from build123d import *

# Parameters (mm, degrees)
SKETCH_1_W          = 4.5
SKETCH_1_H          = 4.5
SKETCH_1_R          = 1.5
EXTRUDE_1_DEPTH     = 2.5
EXTRUDE_1_2_DEPTH   = 2.5
EXTRUDE_1_3_DEPTH   = 2.5
EXTRUDE_1_4_DEPTH   = 2.5
SKETCH_2_W          = 3
SKETCH_2_H          = 65
EXTRUDE_2_DEPTH     = 40
SKETCH_3_W          = 59
SKETCH_3_H          = 40
SKETCH_3_R          = 1
SKETCH_3_R_2        = 1.5
SKETCH_3_W_2        = 32
SKETCH_3_H_2        = 32
EXTRUDE_4_DEPTH     = 2.5
EXTRUDE_5_DEPTH     = 3
EXTRUDE_6_DEPTH     = 3
SKETCH_9_W          = 65
SKETCH_9_H          = 70.660654221
EXTRUDE_8_DEPTH     = 1.8
SKETCH_12_R         = 1
SKETCH_12_W         = 32
SKETCH_12_H         = 32
CUT_EXTRUDE_2_DEPTH = 65
CUT_EXTRUDE_6_DEPTH = 65
SKETCH_14_R         = 1.5
CUT_EXTRUDE_8_DEPTH = 1.8


with BuildPart() as part:
    # Sketch 1 → Extrude 1 (new body)
    with BuildSketch(Plane(origin=(0, 0, 0), x_dir=(1, 0, 0), z_dir=(0, 1, 0))):
        with Locations((-34.75, -30.25)):
            Rectangle(SKETCH_1_W, SKETCH_1_H)
        with Locations(Location((-34.75, -30.25, 0), (0, 0, 270))):
            Circle(SKETCH_1_R, mode=Mode.SUBTRACT)
    extrude(amount=EXTRUDE_1_DEPTH)



with BuildPart() as body_2:
    # Sketch 1 → Extrude 1 2 (new body)
    with BuildSketch(Plane(origin=(0, 0, 0), x_dir=(1, 0, 0), z_dir=(0, 1, 0))):
        with Locations((34.75, -30.25)):
            Rectangle(SKETCH_1_W, SKETCH_1_H)
        with Locations(Location((34.75, -30.25, 0), (0, 0, 270))):
            Circle(SKETCH_1_R, mode=Mode.SUBTRACT)
    extrude(amount=EXTRUDE_1_2_DEPTH)


with BuildPart() as body_3:
    # Sketch 1 → Extrude 1 3 (new body)
    with BuildSketch(Plane(origin=(0, 0, 0), x_dir=(1, 0, 0), z_dir=(0, 1, 0))):
        with Locations((34.75, 30.25)):
            Rectangle(SKETCH_1_W, SKETCH_1_H)
        with Locations(Location((34.75, 30.25, 0), (0, 0, 270))):
            Circle(SKETCH_1_R, mode=Mode.SUBTRACT)
    extrude(amount=EXTRUDE_1_3_DEPTH)


with BuildPart() as body_4:
    # Sketch 1 → Extrude 1 4 (new body)
    with BuildSketch(Plane(origin=(0, 0, 0), x_dir=(1, 0, 0), z_dir=(0, 1, 0))):
        with Locations((-34.75, 30.25)):
            Rectangle(SKETCH_1_W, SKETCH_1_H)
        with Locations(Location((-34.75, 30.25, 0), (0, 0, 270))):
            Circle(SKETCH_1_R, mode=Mode.SUBTRACT)
    extrude(amount=EXTRUDE_1_4_DEPTH)


with BuildPart() as part_1:
    add(part.part)

    add(body_2.part)  # Extrude 2 merges body 2

    add(body_3.part)  # Extrude 2 merges body 3

    add(body_4.part)  # Extrude 2 merges body 4
    # Sketch 2 → Extrude 2 (add)
    with BuildSketch(Plane(origin=(0, 0, 0), x_dir=(-1, 0, 0), z_dir=(0, -1, 0))):
        with Locations((31, 0)):
            Rectangle(SKETCH_2_W, SKETCH_2_H)
        with Locations((-31, 0)):
            Rectangle(SKETCH_2_W, SKETCH_2_H)
    extrude(amount=-EXTRUDE_2_DEPTH)

    # Sketch 5 → Extrude 5 (add)
    with BuildSketch(Plane.ZY.offset(32.5)):
        Polygon((32.5, 40), (-19.677687078, 62.148114133), (-32.543475158, 67.609317163), (-32.5, 40), align=None)
    extrude(amount=-EXTRUDE_5_DEPTH)

    # Sketch 8 → Extrude 6 (add)
    with BuildSketch(Plane(origin=(32.5, 0, 0), x_dir=(0, 0, -1), z_dir=(1, 0, 0))):
        Polygon((-32.5, 40), (32.5, 40), (32.543475158, 67.609317163), align=None)
    extrude(amount=-EXTRUDE_6_DEPTH)



with BuildPart() as body_2_2:
    # Sketch 3 → Extrude 4 (new body)
    with BuildSketch(Plane.XY.offset(32.5)):
        with Locations((0, 20)):
            Rectangle(SKETCH_3_W, SKETCH_3_H)
        with Locations((-17.5, 37.5)):
            Circle(SKETCH_3_R, mode=Mode.SUBTRACT)
        with Locations((17.5, 37.5)):
            Circle(SKETCH_3_R, mode=Mode.SUBTRACT)
        with Locations((17.5, 2.5)):
            Circle(SKETCH_3_R, mode=Mode.SUBTRACT)
        with Locations((-17.5, 2.5)):
            Circle(SKETCH_3_R, mode=Mode.SUBTRACT)
        with Locations((-22.5, 20)):
            Circle(SKETCH_3_R_2, mode=Mode.SUBTRACT)
        with Locations((22.5, 20)):
            Circle(SKETCH_3_R_2, mode=Mode.SUBTRACT)
        with Locations((0, 20)):
            Rectangle(SKETCH_3_W_2, SKETCH_3_H_2, mode=Mode.SUBTRACT)
    extrude(amount=-EXTRUDE_4_DEPTH)


with BuildPart() as part_2:
    add(part_1.part)

    add(body_2_2.part)  # Extrude 8 merges body 2 2
    # Sketch 9 → Extrude 8 (add)
    with BuildSketch(Plane(origin=(0, 45.582439165, 19.348597487), x_dir=(1, 0, 0), z_dir=(0, 0.9205048534524402, 0.3907311284892746))):
        with Locations((0, 21.043164513)):
            Rectangle(SKETCH_9_W, SKETCH_9_H)
    extrude(amount=-EXTRUDE_8_DEPTH)

    # Sketch 12 → Cut-Extrude 2 (cut)
    with BuildSketch(Plane.ZY.offset(32.5)):
        with Locations((-17.5, 37.5)):
            Circle(SKETCH_12_R)
        with Locations((17.5, 37.5)):
            Circle(SKETCH_12_R)
        with Locations((17.5, 2.5)):
            Circle(SKETCH_12_R)
        with Locations((-17.5, 2.5)):
            Circle(SKETCH_12_R)
        with Locations((0, 20)):
            Rectangle(SKETCH_12_W, SKETCH_12_H)
    extrude(amount=-CUT_EXTRUDE_2_DEPTH, mode=Mode.SUBTRACT)

    # Sketch 13 → Cut-Extrude 6 (cut)
    with BuildSketch(Plane(origin=(32.5, 0, 0), x_dir=(0, 0, -1), z_dir=(1, 0, 0))):
        Polygon((32.540393941, 65.652560585), (32.540393941, 67.608009264), (33.246791189, 65.952408427), align=None)
    extrude(amount=-CUT_EXTRUDE_6_DEPTH, mode=Mode.SUBTRACT)


with BuildPart() as body_2_3:
    # of the pieces the cut leaves, the one that is kept (cut_extrude_6_keep)
    add(part_2.part.solids().sort_by_distance((37, 0, -32.5))[0])

    # Sketch 14 → Cut-Extrude 8 (cut)
    with BuildSketch(Plane(origin=(0, 45.582439165, 19.348597487), x_dir=(1, 0, 0), z_dir=(0, 0.92050485345244, 0.39073112848927466))):
        with Locations(Location((18, -3.287162598, 0), (0, 0, 270))):
            Circle(SKETCH_14_R)
        with Locations(Location((16, 20.712837402, 0), (0, 0, 270))):
            Circle(SKETCH_14_R)
        with Locations(Location((18, 44.712837402, 0), (0, 0, 270))):
            Circle(SKETCH_14_R)
        with Locations(Location((-18, -3.287162598, 0), (0, 0, 90))):
            Circle(SKETCH_14_R)
        with Locations(Location((-18, 44.712837402, 0), (0, 0, 90))):
            Circle(SKETCH_14_R)
        with Locations(Location((-23, 20.712837402, 0), (0, 0, 270))):
            Circle(SKETCH_14_R)
    extrude(amount=-CUT_EXTRUDE_8_DEPTH, mode=Mode.SUBTRACT)


solid = body_2_3.part
Geometry: final body of the model. Coordinates: model frame, mm. A direction names the side the tool comes from. Give positions to 0.01 mm unless a question says otherwise; leave off trailing zeros. Write each loop counter-clockwise with the first axis right and the second up, starting at its lowest first coordinate (ties: lowest second). Pieces come first, ordered by that corner, then holes. Notation, with made-up numbers: (17.5, -5.75) -> (69.5, -5.75) arc R25 cw to (69.5, 33.25) -> close; hole circle Ø6 at (75.25, -21.75). An arc over 180 degrees is marked (long way). Answer as a JSON object with one key per item and string values.
1. Cut plane D-D on z = 6.5. Output: boundary loops of the cut face in (x, y), and give its area (3 significant figures).
Ans:
{"outline": "(-32.5, 0) -> (-29.5, 0) -> (-29.5, 4) -> (-32.5, 4) -> close; (-32.5, 36) -> (-29.5, 36) -> (-29.5, 49.08) -> (29.5, 49.08) -> (29.5, 36) -> (32.5, 36) -> (32.5, 51.04) -> (-32.5, 51.04) -> close; (29.5, 0) -> (32.5, 0) -> (32.5, 4) -> (29.5, 4) -> close", "area": "230 mm^2"}
2. Access query for faces 5 (the flat face through (0, 4, 31)), 6 (the flat face through (33, 2.5, -30)), 7 (the flat face through (-29.5, 41, -9)), 8 (the flat face through (31, 20, 16)). Directions: +Z, -Z, +X, -X, +Y, -Y. A direction counts if a zero-diameter tool reaches every point of the face in a straight line with its end or side. Return the directions, or none.
Ans:
{"face 5": "+Z, -Z", "face 6": "+Z, -Z, +X, +Y", "face 7": "-Z, -Y", "face 8": "+X, -X"}
3. Cut plane A-A on x = 12.5. Output: boundary loops of the cut face in (y, z), and give its area (3 significant figures).
Ans:
{"outline": "(0, 30) -> (4, 30) -> (4, 32.5) -> (0, 32.5) -> close; (36, 30) -> (39.11, 30) -> (65.65, -32.54) -> (67.61, -32.54) -> (40, 32.5) -> (36, 32.5) -> close", "area": "144 mm^2"}
4. Mould query, pull axis Z, two halves, no side actions, for faces 1 (the cylindrical face through (-19.265, 62.551, -22.899)), 2 (the flat face through (8, 3, 32.5)), 3 (the cylindrical face through (30.979, 2.8, 18.454)), 4 (the flat face through (-16, 20, 31)). Classes: pulls with the +Z half, pulls with the -Z half, needs draft (parallel to the pull), parting line crosses it, or undercut.
Ans:
{"face 1": "undercut", "face 2": "pulls with the +Z half", "face 3": "undercut", "face 4": "needs draft"}
5. Contact query for flat-ended pins moving along their axis: pin 1 (12 mm diameter, centred on y = 50.5, z = 1.5, fed in from +X); pin 2 (6 mm diameter, centred on x = 8, z = -2, fed in from -Y); pin 3 (8 mm diameter, centred on x = -23.5, z = -19.5, fed in from -Y); pin 4 (1.8 mm diameter, centred on x = -17.5, y = 2.5, fed in from -Z). Output: stop coordinate, or through.
Ans:
{"pin 1": "stops at x = 32.5", "pin 2": "stops at y = 51.42", "pin 3": "stops at y = 58.42", "pin 4": "passes through"}
6. Cut plane B-B on y = 17.5. Output: boundary loops of the cut face in (x, z), and give its area (4 significant figures).
Ans:
{"outline": "(-32.5, -32.5) -> (-29.5, -32.5) -> (-29.5, -16) -> (-32.5, -16) -> close; (-32.5, 16) -> (-29.5, 16) -> (-29.5, 30) -> (-16, 30) -> (-16, 32.5) -> (-32.5, 32.5) -> close; (16, 30) -> (29.5, 30) -> (29.5, 16) -> (32.5, 16) -> (32.5, 32.5) -> (16, 32.5) -> close; (29.5, -32.5) -> (32.5, -32.5) -> (32.5, -16) -> (29.5, -16) -> close", "area": "265.5 mm^2"}
7. Cut plane C-C on x = 30.5. Output: boundary loops of the cut face in (y, z), and give its area (3 significant figures).
Ans:
{"outline": "(0, -32.5) -> (40, -32.5) -> (65.65, -32.54) -> (67.61, -32.54) -> (40, 32.5) -> (0, 32.5) -> close; hole circle Ø2 at (2.5, -17.5); hole circle Ø2 at (2.5, 17.5); hole (4, -16) -> (36, -16) -> (36, 16) -> (4, 16) -> close; hole circle Ø2 at (37.5, -17.5); hole circle Ø2 at (37.5, 17.5)", "area": "2,460 mm^2"}
8. Ray query, probe 1 along X at (y, z) = (36, 21.5); probe 2 along Y at (x, z) = (30.3, 17.5); probe 3 along Y at (x, z) = (30.4, -17.5). Return the intervals inside material, ascending. Write a range as from..to.
Ans:
{"probe 1": "x = -32.5..-29.5, 29.5..32.5", "probe 2": "y = 0..1.5, 3.5..36.5, 38.5..46.37", "probe 3": "y = 0..1.5, 3.5..36.5, 38.5..61.22"}
